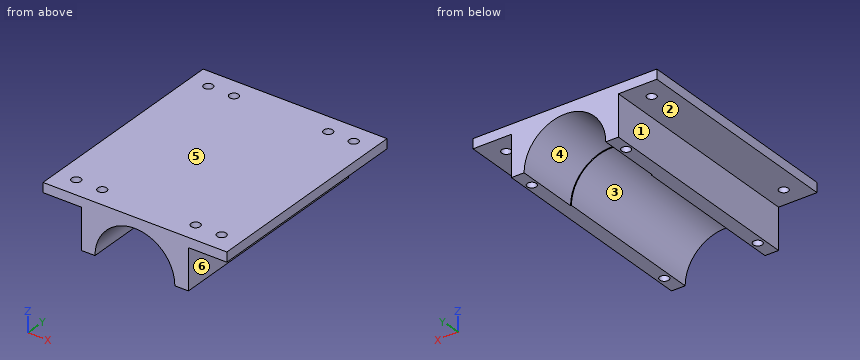
```python
from build123d import *

# Parameters (mm, degrees)
BOSS_EXTRUDE3_DEPTH   = 72.39
BOSS_EXTRUDE4_DEPTH   = 51.39
F_3_0MM_DOWEL_HOLE1_D = 3
F_3_0MM_DOWEL_HOLE2_D = 3
F_3_0MM_DOWEL_HOLE4_D = 3


with BuildPart() as part:
    # Sketch1 → Boss-Extrude3 (new body)
    with BuildSketch(Plane(origin=(0, 0, 0), x_dir=(1, 0, 0), z_dir=(0, 1, 0))):
        with BuildLine():
            Line((-11.1466884, 17.698170271), (-23.8485284, 17.698170271))
            Line((-23.8485284, 17.698170271), (-23.8485284, 14.523170271))
            Line((-23.8485284, 14.523170271), (36.9033116, 14.523170271))
            Line((36.9033116, 14.523170271), (36.9033116, 17.698170271))
            Line((36.9033116, 17.698170271), (24.2033116, 17.698170271))
            Line((24.2033116, 17.698170271), (24.2033116, 31.198170271))
            Line((24.2033116, 31.198170271), (20.025, 31.198170271))
            ThreePointArc((20.025, 31.198170271), (6.525, 17.69817027), (-6.975, 31.198170271))
            Line((-6.975, 31.198170271), (-11.1466884, 31.198170271))
            Line((-11.1466884, 31.198170271), (-11.1466884, 17.698170271))
        make_face()
    extrude(amount=BOSS_EXTRUDE3_DEPTH)

    # Sketch1<13> → Boss-Extrude4 (add)
    with BuildSketch(Plane(origin=(0, 0, 0), x_dir=(1, 0, 0), z_dir=(0, 1, 0))):
        with BuildLine():
            Line((-6.975, 31.198170271), (-6.675, 31.198170271))
            ThreePointArc((-6.675, 31.198170271), (6.525, 17.99817027), (19.725, 31.198170271))
            Line((19.725, 31.198170271), (20.025, 31.198170271))
            ThreePointArc((20.025, 31.198170271), (6.525, 17.69817027), (-6.975, 31.198170271))
        make_face()
    extrude(amount=BOSS_EXTRUDE4_DEPTH)

    # Ø3.0mm Dowel Hole1 (through all)
    with Locations(Plane(origin=(0, 0, -17.698170271), x_dir=(-1, 0, 0), z_dir=(0, 0, -1))):
        with Locations((-30.5533116, 66.04), (-30.5533116, 6.35)):
            Hole(F_3_0MM_DOWEL_HOLE1_D / 2)

    # Ø3.0mm Dowel Hole2 (through all)
    with Locations(Plane(origin=(0, 0, -17.698170271), x_dir=(-1, 0, 0), z_dir=(0, 0, -1))):
        with Locations((17.4985284, 6.35), (17.4985284, 66.04)):
            Hole(F_3_0MM_DOWEL_HOLE2_D / 2)

    # Ø3.0mm Dowel Hole4 (through all)
    with Locations(Plane(origin=(0, 0, -31.198170271), x_dir=(-1, 0, 0), z_dir=(0, 0, -1))):
        with Locations((-22.1133116, 66.04), (9.0566884, 66.04), (8.9066884, 6.35), (-21.9633116, 6.35)):
            Hole(F_3_0MM_DOWEL_HOLE4_D / 2)


solid = part.part
```
The listing builds one solid part. Answer for the finished solid, in the listing's coordinates (mm). Face numbers are marked on the shaded views. A direction names the side the tool comes from. Coordinates: 2 decimals unless noted, no trailing zeros. Order: outer loops, then holes, each group sorted by start corner. A loop starts at its lowest first (then second) coordinate and runs counter-clockwise, first axis right, second up. Notation, with made-up numbers: M 62,36.5 L 87,36.5 A23 cw 87,59.5 Z; hole C -4.75,16 d2. An arc over 180 degrees is marked long. Answer as a JSON object with one key per item and string values. Group by question number.
1. Section B-B on z = -23.75 is taken. Write down the section's boundary in (x, y), then the cut area to 3 significant figures.
2. Determine the mould class of the marked faces 1, 2 and 3 for opening direction X: released by +X, released by -X, zero draft, split by the parting line, or undercut.
3. Section A-A on y = 6.35 is taken. Write down the section's boundary in (x, z) (3 decimals), then the cut area to 3 significant figures.
4. Flat-ended cylindrical pins translate along their axes: P1, Ø6.5, axis at x = -18.5, y = 52.5, coming from the -Z side; P2, Ø1.8, axis at x = 21.96, y = 6.35, coming from the +Z side; P3, Ø8, axis at x = 7, y = 43.5, coming from the -Z side; P4, Ø1, axis at y = 7.5, z = -25, coming from the -X side. Find the tip coordinate at first contact, or state that the pin passes through.
5. Section C-C on x = 21.5 is taken. Write down the section's boundary in (y, z), then the cut area to 3 significant figures.
6. Straight lines are drawn through the part: line 1 (X direction, y = 66, z = -15.75); line 2 (X direction, y = 66.04, z = -21); line 3 (X direction, y = 66.04, z = -19). For each, find the intervals that lie inside material, in ascending order.
7. A tool of negligible diameter and unlimited length cuts with its end or side. For the marked faces 4, 5 and 6, from which of +Z, -Z, +X, -X, +Y, -Y can it reach the whole face along a straight path? Write none if from no direction.
8. Section D-D on y = 66.04 is taken. Write down the section's boundary in (x, z) (3 decimals).
Values follow:
{
 "1": {"outline": "M -11.15,0 L -4.37,0 L -4.37,51.39 L -4.73,51.39 L -4.73,72.39 L -11.15,72.39 Z; M 17.42,0 L 24.2,0 L 24.2,72.39 L 17.78,72.39 L 17.78,51.39 L 17.42,51.39 Z; hole C -9.06,66.04 d3; hole C -8.91,6.35 d3; hole C 21.96,6.35 d3; hole C 22.11,66.04 d3", "area": "938 mm2"},
 "2": {"face 1": "released by -X", "face 2": "zero draft", "face 3": "undercut"},
 "3": {"outline": "M -23.849,-17.698 L -18.999,-17.698 L -18.999,-14.523 L -23.849,-14.523 Z; M -15.999,-17.698 L -11.147,-17.698 L -11.147,-31.198 L -10.407,-31.198 L -10.407,-14.523 L -15.999,-14.523 Z; M -7.407,-31.198 L -6.675,-31.198 A13.2 cw 19.725,-31.198 L 20.463,-31.198 L 20.463,-14.523 L -7.407,-14.523 Z; M 23.463,-31.198 L 24.203,-31.198 L 24.203,-17.698 L 29.053,-17.698 L 29.053,-14.523 L 23.463,-14.523 Z; M 32.053,-17.698 L 36.903,-17.698 L 36.903,-14.523 L 32.053,-14.523 Z", "area": "277 mm2"},
 "4": {"P1": "z = -17.7", "P2": "through", "P3": "z = -18.78", "P4": "x = -11.15"},
 "5": {"outline": "M 0,-31.2 L 4.92,-31.2 L 4.92,-14.52 L 0,-14.52 Z; M 7.78,-31.2 L 64.67,-31.2 L 64.67,-14.52 L 7.78,-14.52 Z; M 67.41,-31.2 L 72.39,-31.2 L 72.39,-14.52 L 67.41,-14.52 Z", "area": "1,110 mm2"},
 "6": {"line 1": "-23.85 to -19, -16 to -10.56, -7.56 to 20.61, 23.61 to 29.05, 32.05 to 36.9", "line 2": "-11.15 to -10.56, -7.56 to -2.32, 15.37 to 20.61, 23.61 to 24.2", "line 3": "-11.15 to -10.56, -7.56 to 0.74, 12.31 to 20.61, 23.61 to 24.2"},
 "7": {"face 4": "-Z, +Y", "face 5": "+Z, +X, -X, +Y, -Y", "face 6": "-Z, +X, +Y, -Y"},
 "8": {"outline": "M -23.849,-17.698 L -18.999,-17.698 L -18.999,-14.523 L -23.849,-14.523 Z; M -15.999,-17.698 L -11.147,-17.698 L -11.147,-31.198 L -10.557,-31.198 L -10.557,-14.523 L -15.999,-14.523 Z; M -7.557,-31.198 L -6.975,-31.198 A13.5 cw 20.025,-31.198 L 20.613,-31.198 L 20.613,-14.523 L -7.557,-14.523 Z; M 23.613,-31.198 L 24.203,-31.198 L 24.203,-17.698 L 29.053,-17.698 L 29.053,-14.523 L 23.613,-14.523 Z; M 32.053,-17.698 L 36.903,-17.698 L 36.903,-14.523 L 32.053,-14.523 Z"}
}
